Verification items for the finished model (mm, model axes). Face numbers are marked on the shaded views. Give positions to 0.01 mm unless a question says otherwise; leave off trailing zeros. Loops run counter-clockwise (first coordinate to the right, second up) from the corner with the lowest first, then second, coordinate; pieces in that order, holes last. Notation, with made-up numbers: (74.25, 15.25) - (92.25, 15.25) arc R13 ccw to (92.25, 34.25) - close; hole circle Ø11 at (77, 57.25). An arc over 180 degrees is marked (long way). Answer in a Markdown table with one row per item.
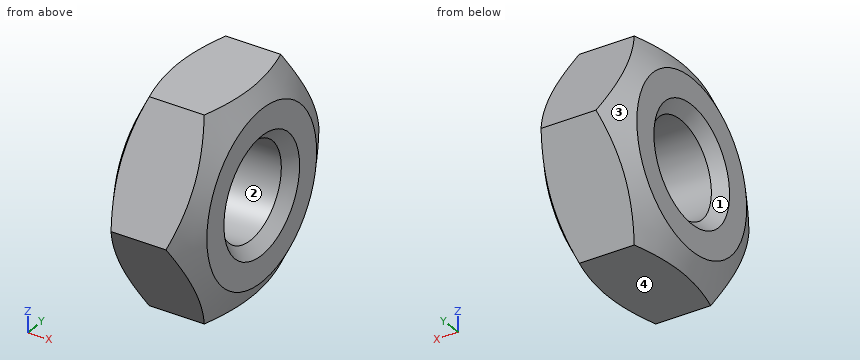
Solid Edge part; units mm, degrees
sketch "Sketch1" plane through (0, 0, 0) normal (0, 0, 1) x (1, 0, 0)
  line L0 (0, 0) -> (0, 4.2)
  line L1 (0, 4.2) -> (3.2, 4.2)
  line L2 (3.2, 4.2) -> (3.2, 0)
  line L3 (3.2, 0) -> (0, 0)
revolve "RevolvedProtrusion1" add sketch "Sketch1" angle 360 about axis through (3.2, 0, 0) along (-1, 0, 0)
sketch "Sketch2" plane through (0, 0, 0) normal (0, 0, 1) x (1, 0, 0)
  line L0 (-1, 7) -> (-1, 2.9)
  line L1 (-1, 2.9) -> (0, 2.9)
  line L2 (0, 2.9) -> (0.7506, 4.2)
  line L3 (0.7506, 4.2) -> (2.4494, 4.2)
  line L4 (2.4494, 4.2) -> (3.2, 2.9)
  line L5 (3.2, 2.9) -> (3.52, 2.9)
  line L6 (3.52, 2.9) -> (3.52, 7)
  line L7 (3.52, 7) -> (-1, 7)
revolve "RevolvedCutout1" cut sketch "Sketch2" angle 360 about axis through (3.2, 0, 0) along (-1, 0, 0)
sketch "Sketch3" plane through (0, 0, 0) normal (0, 0, 1) x (1, 0, 0)
  line L0 (0, 0) -> (0, 2)
  line L1 (0, 2) -> (0.379, 1.621)
  line L2 (0.379, 1.621) -> (2.821, 1.621)
  line L3 (2.821, 1.621) -> (3.2, 2)
  line L4 (3.2, 2) -> (3.2, 0)
  line L5 (3.2, 0) -> (0, 0)
revolve "RevolvedCutout2" cut sketch "Sketch3" angle 360 about axis through (3.2, 0, 0) along (-1, 0, 0)
sketch "Sketch4" plane through (0, 0, 0) normal (1, 0, 0) x (0, 1, 0)
  line L0 (14, 14) -> (-14, 14)
  line L1 (-14, 14) -> (-14, -14)
  line L2 (-14, -14) -> (14, -14)
  line L3 (14, -14) -> (14, 14)
  line L4 (-2.0207, 3.5) -> (-4.0415, 0)
  line L5 (-4.0415, 0) -> (-2.0207, -3.5)
  line L6 (-2.0207, -3.5) -> (2.0207, -3.5)
  line L7 (2.0207, -3.5) -> (4.0415, 0)
  line L8 (4.0415, 0) -> (2.0207, 3.5)
  line L9 (2.0207, 3.5) -> (-2.0207, 3.5)
extrude "ExtrudedCutout_1" cut sketch "Sketch4" against normal blind 4.2 and the other way blind 4.2
properties part number "Hexagon nut DIN 934 M4 01100.040.001(High)"
Q1. Go/stop test with a flat-tipped pin: P1, Ø3.5, axis at y = 0, z = 0, coming from the -X side. Record where the tip stops, or that it passes through.
Completed:
| item | result |
|---|---|
| P1 | x = 0.25 |
Q2. Draft check along Y on the marked faces 1, 2, 3 and 4. Enter one of: +Y half, -Y half, draft (parallel to the pull), parting line (faces both ways), or undercut.
Completed:
| item | result |
|---|---|
| face 1 | undercut |
| face 2 | undercut |
| face 3 | parting line |
| face 4 | draft |
Q3. Thickness scan on line 1 (Z direction, x = 1.55, y = 0); line 2 (Z direction, x = 2.95, y = 1.5); line 3 (Y direction, x = 0.6, z = -0.75). Record the ranges inside material, lowest first.
Completed:
| item | result |
|---|---|
| line 1 | -3.5 to -1.62, 1.62 to 3.5 |
| line 2 | -2.98 to -0.9, 0.9 to 2.98 |
| line 3 | -3.61 to -1.44, 1.44 to 3.61 |
Q4. Sectioned sample at A-A (y = 0). Record the cut outline in (x, z), and give its area (3 significant figures).
Completed:
| item | result |
|---|---|
| outline | (0, -2.9) - (0.35, -3.5) - (2.85, -3.5) - (3.2, -2.9) - (3.2, -2) - (2.82, -1.62) - (0.38, -1.62) - (0, -2) - close; (0, 2) - (0.38, 1.62) - (2.82, 1.62) - (3.2, 2) - (3.2, 2.9) - (2.85, 3.5) - (0.35, 3.5) - (0, 2.9) - close |
| area | 11.3 mm^2 |
Q5. Sectioned sample at B-B (x = 2.3). Record the cut outline in (y, z), and give its area (3 significant figures).
Completed:
| item | result |
|---|---|
| outline | (-4.04, 0) - (-2.02, -3.5) - (2.02, -3.5) - (4.04, 0) - (2.02, 3.5) - (-2.02, 3.5) - close; hole circle Ø3.24 at (0, 0) |
| area | 34.2 mm^2 |
